from build123d import *

# Parameters (mm, degrees)
F0_R            = 25
F1_DEPTH        = 40
F2_SIZE2        = 5
F2_SIZE         = 25
F7_COPIES_COUNT = 8
F8_R            = 15
F9_DEPTH        = 31
F10_R           = 10
F11_DEPTH       = 198


# Not quite as in the source:
# - a pattern or mirror of a feature is missing from the dataset's text; its kind, count and spacing are read off the source's solid


with BuildPart() as f1:
    # F0 (on Front) → F1 (new body)
    with BuildSketch(Plane.XZ):
        Circle(F0_R)
    extrude(amount=F1_DEPTH)

    # F2
    f2_edges = [f1.edges().sort_by_distance(p)[0] for p in [
        (-25, 0, 0),
    ]]
    f2_side = f1.faces().sort_by_distance((-25, -20, 0))[0]
    chamfer(f2_edges, length=F2_SIZE, length2=F2_SIZE2, reference=f2_side)

    # F4 (on Front) → F7 section 0
    with BuildSketch(Plane.XZ):
        Polygon((8, -38), (2, -12), (-2, -12), (-8, -38), align=None)
    # F5 (on offset) → F7 section 1
    with BuildSketch(Plane.XZ.offset(25)):
        Polygon((8, -38), (2, -12), (-2, -12), (-8, -38), align=None)
    f7 = loft(mode=Mode.SUBTRACT)

    # F7_copies: F7 ×8 about axis
    f7_copies_axis = Axis((0, 0, 0), (0, 1, 0))
    for i in range(1, F7_COPIES_COUNT):
        add(f7.rotate(f7_copies_axis, i * 360 / F7_COPIES_COUNT), mode=Mode.SUBTRACT)

    # F8 (on face) → F9 (join)
    with BuildSketch(Plane.XZ.offset(40)):
        Circle(F8_R)
    extrude(amount=F9_DEPTH)

    # F10 (on face) → F11 (join)
    with BuildSketch(Plane.XZ.offset(71)):
        Circle(F10_R)
    extrude(amount=F11_DEPTH)


solid = f1.part
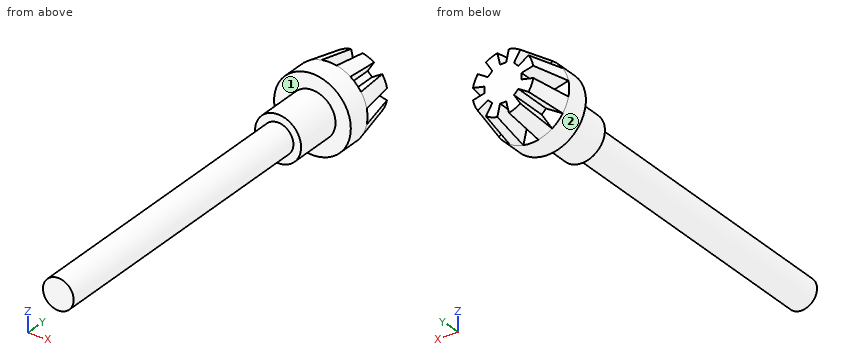
Input: part model. Units: mm. Frame: model coordinates. Face numbers are marked on the shaded views. A direction names the side the tool comes from. Coordinates: 2 decimals unless noted, no trailing zeros. Order: outer loops, then holes, each group sorted by start corner. A loop starts at its lowest first (then second) coordinate and runs counter-clockwise, first axis right, second up. Notation, with made-up numbers: M -34.5,10 L -14.5,10 A19 ccw -14.5,25 Z; hole C 43,68.5 d8. An arc over 180 degrees is marked long. Answer as CSV lines item,"result".
1. First-contact query: P1, Ø8, axis at x = -1.5, z = 18.5, coming from the +Y side; P2, Ø8, axis at x = 2.5, y = -102, coming from the +Z side; P3, Ø4, axis at x = 14.5, z = -16.5, coming from the +Y side; P4, Ø10, axis at y = -29.5, z = -9, coming from the +X side. Flat tips, straight axial feed; report the tip coordinate or a pass-through.
Reported:
P1,"y = 0"
P2,"z = 10"
P3,"y = -25"
P4,"x = 24.68"
2. Section A-A (y = -134.5). Return the cut outline in (x, z).
Reported:
outline,"C 0,0 d20"
3. Material intervals for line 1 (Z direction, x = 9, y = -16); line 2 (Z direction, x = -1.5, y = -172); line 3 (Z direction, x = -7.5, y = -19), sorted ascending. Write a range as from..to.
Reported:
line 1,"-21.38..-12.99, -7.97..7.97, 12.99..21.38"
line 2,"-9.89..9.89"
line 3,"-22.59..-10.59, -9.47..9.47, 10.59..22.59"
4. Access query for the marked faces 1 and 2. Directions: +Z, -Z, +X, -X, +Y, -Y. A direction counts if a zero-diameter tool reaches every point of the face in a straight line with its end or side. Return the directions, or none.
Reported:
face 1,"-Y"
face 2,"+Y, -Y"
